```python
from build123d import *

# Parameters (mm, degrees)
SKETCH2_R          = 5.7
CUT_EXTRUDE1_DEPTH = 17.78
SKETCH3_R          = 10.717201778
CUT_EXTRUDE2_DEPTH = 2.032
CUT_EXTRUDE3_DEPTH = 2.032


with BuildPart() as part:
    # Sketch1 → Revolve1 (revolve)
    with BuildSketch(Plane(origin=(0, 0, 0), x_dir=(0, 0, -1), z_dir=(1, 0, 0)), mode=Mode.PRIVATE) as revolve1_sk:
        Polygon((0, 0), (0, 15.800000023), (2, 15.800000023), (2, 15.600000023), (8.5, 15.600000023), (8.5, 12.5), (15, 12.5), (26, 9), (26, 0), align=None)
    revolve(revolve1_sk.sketch.rotate(Axis((0, 0, 0), (0, 0, 1)), 90), axis=Axis((0, 0, 0), (0, 0, 1)))

    # Sketch2 → Cut-Extrude1 (cut)
    with BuildSketch(Plane(origin=(0, 0, -26), x_dir=(-1, 0, 0), z_dir=(0, 0, -1))):
        Circle(SKETCH2_R)
    extrude(amount=-CUT_EXTRUDE1_DEPTH, mode=Mode.SUBTRACT)

    # Sketch3 → Cut-Extrude2 (cut)
    with BuildSketch(Plane.XY):
        Circle(SKETCH3_R)
        Polygon((4.561067127, 7.9), (-4.561067127, 7.9), (-9.122134253, 0), (-4.561067127, -7.9), (4.561067127, -7.9), (9.122134253, 0), align=None, mode=Mode.SUBTRACT)
    extrude(amount=-CUT_EXTRUDE2_DEPTH, mode=Mode.SUBTRACT)

    # Sketch4 → Cut-Revolve1 (revolve, cut)
    with BuildSketch(Plane(origin=(0, 0, 0), x_dir=(1, 0, 0), z_dir=(0, 1, 0)), mode=Mode.PRIVATE) as cut_revolve1_sk:
        with BuildLine():
            Line((-9.122134253, 1.016), (-9.122134253, 0))
            Line((-9.122134253, 0), (-7.217734963, 0))
            ThreePointArc((-7.217734963, 0), (-8.258276499, 0.342411186), (-9.122134253, 1.016))
        make_face()
    revolve(cut_revolve1_sk.sketch.rotate(Axis((0, 0, 0), (0, 0, -1)), 180), axis=Axis((0, 0, 0), (0, 0, -1)), mode=Mode.SUBTRACT)

    # Sketch5 → Cut-Extrude3 (cut)
    with BuildSketch(Plane.XY):
        Polygon((0, 3.648853701), (-3.16, 1.824426851), (-3.16, -1.824426851), (0, -3.648853701), (3.16, -1.824426851), (3.16, 1.824426851), align=None)
    extrude(amount=-CUT_EXTRUDE3_DEPTH, mode=Mode.SUBTRACT)


solid = part.part
```
Read the model definition and answer for the solid it produces. Units are mm, in the model's axes. A direction names the side the tool comes from. Round coordinates to 2 decimals unless told otherwise and drop trailing zeros. Write each loop counter-clockwise with the first axis right and the second up, starting at its lowest first coordinate (ties: lowest second). Pieces come first, ordered by that corner, then holes. Notation, with made-up numbers: M 19,55 L 36,55 A21 ccw 36,79 Z; hole C 88.25,42 d3. An arc over 180 degrees is marked long. One line per item, written item: value.
Q1. Which of the six approach directions +Z, -Z, +X, -X, +Y, -Y give full straight-line access (tool end or side, diameter ignored) to faces 4 (the flat face through (0, 7.9, -1)), 5 (the cylindrical face through (-11.923, -3.755, -11.796)), 6 (the flat face through (0, 6, -26))?
Data:
face 4: +Z
face 5: -Z
face 6: -Z, +X, -X, +Y, -Y
Q2. Find section A-A on z = -9.25. Write down the section's boundary in (x, y).
Data:
outline: C 0,0 d25; hole C 0,0 d11.4
Q3. For a pull along X with two mould halves and no side action, classify faces 1 (the cylindrical face through (4.5, -3.5, -17.2)), 2 (the cylindrical face through (11.5, -10.54, -5.3)), 3 (the flat face through (2, 3, 0)) as +X half, -X half, draft (parallel to the pull), parting line (faces both ways), or undercut.
Data:
face 1: undercut
face 2: parting line
face 3: draft
Q4. Straight lines are drawn through the part: line 1 (Y direction, x = 0, z = -0.65); line 2 (Y direction, x = 0, z = -11.75); line 3 (Z direction, x = -1.5, y = 2). For each, find the intervals that lie inside material, in ascending order. Write a range as [from, to].
Data:
line 1: [-15.8, -10.72], [-7.9, -3.65], [3.65, 7.9], [10.72, 15.8]
line 2: [-12.5, -5.7], [5.7, 12.5]
line 3: [-8.22, -2.03]
Q5. Flat-ended cylindrical pins translate along their axes: pin 1 Ø8 at (x, z) = (-7.5, -6.5) entering from +Y; pin 2 Ø2 at (x, z) = (-1.5, -18.5) entering from +Y; pin 3 Ø6 at (y, z) = (11.5, -21) entering from -X. Find the tip coordinate at first contact, or state that the pin passes through.
Data:
pin 1: y = 15.2
pin 2: y = 11.63
pin 3: x = -6.62
Q6. Find section B-B on z = -15.5. Write down the section's boundary in (x, y), plus the area to 3 significant figures.
Data:
outline: C 0,0 d24.68; hole C 0,0 d11.4
area: 376 mm2
